```python
from build123d import *

# Parameters (mm, degrees)
CROQUIS1_W                   = 400
CROQUIS1_H                   = 250
SALIENTE_EXTRUIR1_DEPTH      = 50
CORTAR_EXTRUIR1_DEPTH        = 30
TALADRO1_D                   = 14
TALADRO1_DEPTH               = 49.877349569
TALADRO1_CBORE_D             = 21
TALADRO1_CBORE_DEPTH         = 14
MATRIZL1_COUNT               = 7
MATRIZL1_PITCH               = 30
SIMETR_A1_COPY_1_D           = 14
SIMETR_A1_COPY_1_DEPTH       = 49.877349569
SIMETR_A1_COPY_1_CBORE_D     = 21
SIMETR_A1_COPY_1_CBORE_DEPTH = 14
SIMETR_A1_COPY_2_D           = 14
SIMETR_A1_COPY_2_DEPTH       = 49.877349569
SIMETR_A1_COPY_2_CBORE_D     = 21
SIMETR_A1_COPY_2_CBORE_DEPTH = 14
SIMETR_A1_COPY_3_D           = 14
SIMETR_A1_COPY_3_DEPTH       = 49.877349569
SIMETR_A1_COPY_3_CBORE_D     = 21
SIMETR_A1_COPY_3_CBORE_DEPTH = 14
SIMETR_A1_COPY_4_D           = 14
SIMETR_A1_COPY_4_DEPTH       = 49.877349569
SIMETR_A1_COPY_4_CBORE_D     = 21
SIMETR_A1_COPY_4_CBORE_DEPTH = 14
SIMETR_A1_COPY_5_D           = 14
SIMETR_A1_COPY_5_DEPTH       = 49.877349569
SIMETR_A1_COPY_5_CBORE_D     = 21
SIMETR_A1_COPY_5_CBORE_DEPTH = 14
SIMETR_A1_COPY_6_D           = 14
SIMETR_A1_COPY_6_DEPTH       = 49.877349569
SIMETR_A1_COPY_6_CBORE_D     = 21
SIMETR_A1_COPY_6_CBORE_DEPTH = 14


with BuildPart() as part:
    # Croquis1 → Saliente-Extruir1 (new body)
    with BuildSketch(Plane(origin=(0, 0, 0), x_dir=(1, 0, 0), z_dir=(0, 1, 0))):
        Rectangle(CROQUIS1_W, CROQUIS1_H)
        with BuildLine():
            Line((-100, 75), (100, 75))
            ThreePointArc((100, 75), (117.67766953, 67.67766953), (125, 50))
            Line((125, 50), (125, -50))
            ThreePointArc((125, -50), (117.67766953, -67.67766953), (100, -75))
            Line((100, -75), (-100, -75))
            ThreePointArc((-100, -75), (-117.67766953, -67.67766953), (-125, -50))
            Line((-125, -50), (-125, 50))
            ThreePointArc((-125, 50), (-117.67766953, 67.67766953), (-100, 75))
        make_face(mode=Mode.SUBTRACT)
    extrude(amount=SALIENTE_EXTRUIR1_DEPTH)

    # Croquis2 → Cortar-Extruir1 (cut)
    with BuildSketch(Plane(origin=(0, 50, 0), x_dir=(1, 0, 0), z_dir=(0, 1, 0))):
        with BuildLine():
            Line((-135, 95), (135, 95))
            ThreePointArc((135, 95), (145.606601718, 90.606601718), (150, 80))
            Line((150, 80), (150, -80))
            ThreePointArc((150, -80), (145.606601718, -90.606601718), (135, -95))
            Line((135, -95), (-135, -95))
            ThreePointArc((-135, -95), (-145.606601718, -90.606601718), (-150, -80))
            Line((-150, -80), (-150, 80))
            ThreePointArc((-150, 80), (-145.606601718, 90.606601718), (-135, 95))
        make_face()
    extrude(amount=-CORTAR_EXTRUIR1_DEPTH, mode=Mode.SUBTRACT)

    # Taladro1
    with Locations(Plane(origin=(0, 50, 0), x_dir=(1, 0, 0), z_dir=(0, 1, 0))):
        with Locations((-175, 100)):
            taladro1 = CounterBoreHole(TALADRO1_D / 2, TALADRO1_CBORE_D / 2, TALADRO1_CBORE_DEPTH, depth=TALADRO1_DEPTH)

    # MatrizL1: Taladro1 ×7
    with Locations(*[(0, 0, i * MATRIZL1_PITCH) for i in range(1, MATRIZL1_COUNT)]):
        add(taladro1, mode=Mode.SUBTRACT)

    # Simetría1: Taladro1 across plane
    add(taladro1.mirror(Plane(origin=(0, 0, 0), x_dir=(0, 0, 1), z_dir=(1, 0, 0))), mode=Mode.SUBTRACT)

    # Simetría1 copy 1
    with Locations(Plane(origin=(0, 50, 30), x_dir=(-1, 0, 0), z_dir=(0, 1, 0))):
        with Locations((-175, -100)):
            CounterBoreHole(SIMETR_A1_COPY_1_D / 2, SIMETR_A1_COPY_1_CBORE_D / 2, SIMETR_A1_COPY_1_CBORE_DEPTH, depth=SIMETR_A1_COPY_1_DEPTH)

    # Simetría1 copy 2
    with Locations(Plane(origin=(0, 50, 60), x_dir=(-1, 0, 0), z_dir=(0, 1, 0))):
        with Locations((-175, -100)):
            CounterBoreHole(SIMETR_A1_COPY_2_D / 2, SIMETR_A1_COPY_2_CBORE_D / 2, SIMETR_A1_COPY_2_CBORE_DEPTH, depth=SIMETR_A1_COPY_2_DEPTH)

    # Simetría1 copy 3
    with Locations(Plane(origin=(0, 50, 90), x_dir=(-1, 0, 0), z_dir=(0, 1, 0))):
        with Locations((-175, -100)):
            CounterBoreHole(SIMETR_A1_COPY_3_D / 2, SIMETR_A1_COPY_3_CBORE_D / 2, SIMETR_A1_COPY_3_CBORE_DEPTH, depth=SIMETR_A1_COPY_3_DEPTH)

    # Simetría1 copy 4
    with Locations(Plane(origin=(0, 50, 120), x_dir=(-1, 0, 0), z_dir=(0, 1, 0))):
        with Locations((-175, -100)):
            CounterBoreHole(SIMETR_A1_COPY_4_D / 2, SIMETR_A1_COPY_4_CBORE_D / 2, SIMETR_A1_COPY_4_CBORE_DEPTH, depth=SIMETR_A1_COPY_4_DEPTH)

    # Simetría1 copy 5
    with Locations(Plane(origin=(0, 50, 150), x_dir=(-1, 0, 0), z_dir=(0, 1, 0))):
        with Locations((-175, -100)):
            CounterBoreHole(SIMETR_A1_COPY_5_D / 2, SIMETR_A1_COPY_5_CBORE_D / 2, SIMETR_A1_COPY_5_CBORE_DEPTH, depth=SIMETR_A1_COPY_5_DEPTH)

    # Simetría1 copy 6
    with Locations(Plane(origin=(0, 50, 180), x_dir=(-1, 0, 0), z_dir=(0, 1, 0))):
        with Locations((-175, -100)):
            CounterBoreHole(SIMETR_A1_COPY_6_D / 2, SIMETR_A1_COPY_6_CBORE_D / 2, SIMETR_A1_COPY_6_CBORE_DEPTH, depth=SIMETR_A1_COPY_6_DEPTH)


solid = part.part
```
Model file for the job. Use its own axes, mm. A direction names the side the tool comes from. Give positions to 0.01 mm unless a question says otherwise; leave off trailing zeros. Write each loop counter-clockwise with the first axis right and the second up, starting at its lowest first coordinate (ties: lowest second). Pieces come first, ordered by that corner, then holes. Notation, with made-up numbers: M 16.25,52 L 22.25,52 A14 cw 22.25,71 Z; hole C 57,69 d7. An arc over 180 degrees is marked long. Use a Markdown table: item, result.
1) Cut at D-D (x = -142). List the corners of the cut face in (y, z), and give its area (3 significant figures).
Responses:
| item | result |
|---|---|
| outline | M 0,-125 L 50,-125 L 50,-93.27 L 20,-93.27 L 20,93.27 L 50,93.27 L 50,125 L 0,125 Z |
| area | 6,900 mm2 |
2) Cut at B-B (x = -64). List the corners of the cut face in (y, z), and give its area (3 significant figures).
Responses:
| item | result |
|---|---|
| outline | M 0,-125 L 50,-125 L 50,-95 L 20,-95 L 20,-75 L 0,-75 Z; M 0,75 L 20,75 L 20,95 L 50,95 L 50,125 L 0,125 Z |
| area | 3,800 mm2 |
3) Pull direction Z, two halves, no side cores. Call faces 1 (the flat face through (-173, 36, 57)), 2 (the flat face through (200, 25, 2)): +Z half, -Z half, draft (parallel to the pull), parting line (faces both ways), or undercut.
Responses:
| item | result |
|---|---|
| face 1 | undercut |
| face 2 | draft |
4) Cut at A-A (y = 12.5). Give the number of separate pieces and of enclosed holes in the cut face, and give its area (3 significant figures).
Responses:
| item | result |
|---|---|
| separate pieces | 1 |
| enclosed holes | 15 |
| area | 60,900 mm2 |
5) Pin check, flat tips, straight feed: pin 1 (7 mm diameter, centred on x = 178, z = -10, fed in from +Y); pin 2 (8 mm diameter, centred on x = -46, z = -82.5, fed in from +Y); pin 3 (1 mm diameter, centred on x = -124, z = 42.5, fed in from +Y); pin 4 (6.5 mm diameter, centred on x = 178, z = -44, fed in from +Y). Stop position of each tip, or through.
Responses:
| item | result |
|---|---|
| pin 1 | stops at y = 0.12 |
| pin 2 | stops at y = 20 |
| pin 3 | passes through |
| pin 4 | stops at y = 36 |
6) Cut at C-C (z = -40). List the corners of the cut face in (x, y), and give its area (3 significant figures).
Responses:
| item | result |
|---|---|
| outline | M -200,0 L -125,0 L -125,20 L -150,20 L -150,50 L -164.5,50 L -164.5,36 L -168,36 L -168,0.12 L -182,0.12 L -182,36 L -185.5,36 L -185.5,50 L -200,50 Z; M 125,0 L 200,0 L 200,50 L 185.5,50 L 185.5,36 L 182,36 L 182,0.12 L 168,0.12 L 168,36 L 164.5,36 L 164.5,50 L 150,50 L 150,20 L 125,20 Z |
| area | 4,410 mm2 |
7) Drill centre lines: line 1 (X direction, y = 42.5, z = -100); line 2 (X direction, y = 16, z = -100); line 3 (Z direction, x = -15, y = 40). Where is each one in solid material? Low to high. Write a range as from..to.
Responses:
| item | result |
|---|---|
| line 1 | x = -200..-185.5, -164.5..164.5, 185.5..200 |
| line 2 | x = -200..-182, -168..168, 182..200 |
| line 3 | z = -125..-95, 95..125 |
8) Tool access for faces 3 (the cylindrical face through (-165, 43.1, -43.2)), 4 (the flat face through (-1, 10, -75)): list every direction of +Z, -Z, +X, -X, +Y, -Y with a clear straight run to the whole face (end or side of a thin tool).
Responses:
| item | result |
|---|---|
| face 3 | +Y |
| face 4 | +Y, -Y |
